Autodesk Inventor part; units mm, degrees
ref_plane "YZ Plane" through (0, 0, 0) normal (1, 0, 0) x (0, 1, 0)
ref_plane "XZ Plane" through (0, 0, 0) normal (0, 1, 0) x (-1, 0, 0)
ref_plane "XY Plane" through (0, 0, 0) normal (0, 0, 1) x (1, 0, 0)
sketch "Sketch1" plane through (0, 0, 0) normal (0, 1, 0) x (-1, 0, 0)
  line L0 (-3.175, -3.175) -> (3.175, -3.175)
  line L1 (3.175, -3.175) -> (3.175, 3.175)
  line L2 (3.175, 3.175) -> (-3.175, 3.175)
  line L3 (-3.175, 3.175) -> (-3.175, -3.175)
  line L4 (-3.175, -3.175) -> (3.175, 3.175) construction
  line L5 (3.175, -3.175) -> (-3.175, 3.175) construction
  point P0 (0, 0)
  dimension "d0" = 6.35
  dimension "d1" = 6.35
extrude "Extrusion1" add sketch "Sketch1" along normal blind 120.65
fillet "Fillet1" radius 1.5875 4 edges at (3.175, 60.325, 3.175) (3.175, 60.325, -3.175) (-3.175, 60.325, -3.175) (-3.175, 60.325, 3.175)
fillet "Fillet2" radius 0.7937 16 edges at (2.71, 120.65, -2.71) (0, 120.65, -3.175) (-2.71, 120.65, -2.71) (-3.175, 120.65, 0) (-2.71, 120.65, 2.71) (0, 120.65, 3.175) (2.71, 120.65, 2.71) (3.175, 120.65, 0) (2.71, 0, -2.71) (0, 0, -3.175) (-2.71, 0, -2.71) (-3.175, 0, 0) (-2.71, 0, 2.71) (0, 0, 3.175) (2.71, 0, 2.71) (3.175, 0, 0)
sketch "Sketch2" plane through (-1.5875, 0.7937, 3.175) normal (0, 0, 1) x (1, 0, 0)
  circle A0 centre (1.5875, 5.5563) radius 1.9844
  line L0 (0, -0.7937) -> (3.175, -0.7937)
  point P0 (1.5875, -0.7937)
  dimension "d6" = 3.9688
  dimension "d7" = 6.35
extrude "Extrusion2" cut sketch "Sketch2" against normal blind 120.65
sketch "Sketch3" plane through (3.175, 0.7937, -1.5875) normal (1, 0, 0) x (0, 0, -1)
  circle A0 centre (-1.5875, 116.6812) radius 1.9844
  line L0 (0, 119.8562) -> (-3.175, 119.8562)
  line L1 (1.5875, 6.7469) -> (1.5875, 119.0625)
  point P0 (-1.5875, -0.7937)
  dimension "d10" = 3.9688
  dimension "d11" = 3.175
  dimension "d12" = 3.175
extrude "Extrusion3" cut sketch "Sketch3" against normal blind 120.65
sketch "Sketch4" plane through (-1.5875, 119.8562, 3.175) normal (0, 0, 1) x (1, 0, 0)
  arc A0 (3.175, -112.3156) -> (0, -112.3156) centre (1.5875, -113.5062) ccw
  circle A1 centre (1.5875, -75.4062) radius 1.9844
  point P0 (1.5875, -119.8562)
  dimension "d15" = 3.9688
  dimension "d16" = 38.1
extrude "Extrusion4" cut sketch "Sketch4" against normal blind 120.65
properties part number "support beam" material "Stainless Steel"
The model under review builds one solid part; all positions refer to its coordinate system, in mm. Round coordinates to 2 decimals unless told otherwise and drop trailing zeros. Order: outer loops, then holes, each group sorted by start corner. A loop starts at its lowest first (then second) coordinate and runs counter-clockwise, first axis right, second up. Notation, with made-up numbers: (5.5, 79) -> (43.5, 79) arc R21 ccw to (43.5, 108) -> close; hole circle Ø5 at (16, 4). An arc over 180 degrees is marked (long way). Use CSV: the item, a comma, the result in double quotes. Start each with the question number.
(1) Consider section C-C on y = 44.45. Write out the cut boundary in (x, z) (1 decimal).
(2) Consider section B-B on x = 0. Write out the cut boundary in (y, z) (3 decimals), and give its area (3 significant figures).
(3) Wall thickness on probe 1 along Y at (x, z) = (1.5, -2.75); probe 2 along X at (y, z) = (44.45, -0.75) (3 decimals); probe 3 along X at (y, z) = (98, -1.75): over which ranges is each line inside the solid? List them lowest first. Write a range as from..to.
(4) Mouldability with a two-part tool opening along Y and no side actions: class faces 1 (the face through (0, 25, -3.175)), 2 (the face through (0, 0, 0)), 3 (the face through (-0.258, 46.418, 0.044)) as pulls with the +Y half, pulls with the -Y half, needs draft (parallel to the pull), parting line crosses it, or undercut.
(5) Consider section A-A on z = 0. State how many separate pieces and enclosed holes the cut face has, and give its area (3 significant figures).
(6) Insertion check: pin 1 (3.5 mm diameter, centred on x = 0, y = 6.35, fed in from +Z). The pin has a flat end and moves straight along its axis. Give the tip position at first contact, or say it passes through.
Responses:
1,outline,"(-3.2, -1.6) arc R1.6 ccw to (-2, -3.1) -> (-2, 3.1) arc R1.6 ccw to (-3.2, 1.6) -> close; (2, -3.1) arc R1.6 ccw to (3.2, -1.6) -> (3.2, 1.6) arc R1.6 ccw to (2, 3.1) -> close"
2,outline,"(0, -2.381) arc R0.794 ccw to (0.794, -3.175) -> (4.366, -3.175) -> (4.366, 3.175) -> (0.794, 3.175) arc R0.794 ccw to (0, 2.381) -> close; (8.334, -3.175) -> (42.466, -3.175) -> (42.466, 3.175) -> (8.334, 3.175) -> close; (46.434, -3.175) -> (119.856, -3.175) arc R0.794 ccw to (120.65, -2.381) -> (120.65, 2.381) arc R0.794 ccw to (119.856, 3.175) -> (46.434, 3.175) -> close; hole circle Ø3.969 at (117.475, 0)"
2,area,"703 mm²"
3,probe 1,"0.09..5.05, 7.65..43.15, 45.75..120.56"
3,probe 2,"-3.175..-1.984, 1.984..3.175"
3,probe 3,"-3.17..3.17"
4,face 1,"needs draft"
4,face 2,"pulls with the -Y half"
4,face 3,"undercut"
5,separate pieces,"2"
5,enclosed holes,"2"
5,area,"716 mm²"
6,pin 1,"through"
